```python
from build123d import *

# Parameters (mm, degrees)
EXTRUDE_1_DEPTH = 5
SKETCH_2_R      = 2.5
EXTRUDE_2_DEPTH = 8
SKETCH_3_R      = 3
EXTRUDE_3_DEPTH = 15
SKETCH_5_R      = 3.5
EXTRUDE_4_DEPTH = 2
SKETCH_4_W      = 0.25
SKETCH_4_H      = 0.7
SKETCH_4_W_2    = 1.323985747
SKETCH_4_H_2    = 1
CHAMFER_1_SIZE  = 0.2


with BuildPart() as part:
    # 草图1 → 拉伸1 (new body)
    with BuildSketch(Plane.XY):
        with BuildLine():
            Line((-2.633913438, 4.25), (2.633913438, 4.25))
            ThreePointArc((2.633913438, 4.25), (4.982386472, 0.419314968), (3.307189139, -3.75))
            Line((3.307189139, -3.75), (-3.307189139, -3.75))
            ThreePointArc((-3.307189139, -3.75), (-4.982386472, 0.419314968), (-2.633913438, 4.25))
        make_face()
    extrude(amount=EXTRUDE_1_DEPTH)

    # 草图2 → 拉伸2 (add)
    with BuildSketch(Plane.XY.offset(5)):
        Circle(SKETCH_2_R)
    extrude(amount=EXTRUDE_2_DEPTH)

    # 草图3 → 拉伸3 (add)
    with BuildSketch(Plane(origin=(0, 0, 0), x_dir=(-1, 0, 0), z_dir=(0, 0, -1))):
        with Locations(Location((0, 0, 0), (0, 0, 180))):
            Circle(SKETCH_3_R)
    extrude(amount=EXTRUDE_3_DEPTH)

    # 草图5 → 拉伸4 (add)
    with BuildSketch(Plane(origin=(0, 0, 0), x_dir=(-1, 0, 0), z_dir=(0, 0, -1))):
        with Locations(Location((0, 0, 0), (0, 0, 180))):
            Circle(SKETCH_5_R)
    extrude(amount=EXTRUDE_4_DEPTH)

    # 草图4 → 切除-旋转1 (revolve, cut)
    with BuildSketch(Plane(origin=(0, 0, 0), x_dir=(1, 0, 0), z_dir=(0, 1, 0))):
        with Locations((-2.875, 13.55)):
            Rectangle(SKETCH_4_W, SKETCH_4_H)
        with Locations((-2.661992874, -5.5)):
            Rectangle(SKETCH_4_W_2, SKETCH_4_H_2)
    revolve(axis=Axis((0, 0, -15), (0, 0, 1)), mode=Mode.SUBTRACT)

    # 倒角1
    chamfer_1_edges = [part.edges().sort_by_distance(p)[0] for p in [
        (-2.5, 0, 13),
        (-3, 0, -15),
    ]]
    chamfer(chamfer_1_edges, length=CHAMFER_1_SIZE)


solid = part.part
```
Read the model definition and answer for the solid it produces. Units are mm, in the model's axes. A direction names the side the tool comes from. Round coordinates to 2 decimals unless told otherwise and drop trailing zeros. Write each loop counter-clockwise with the first axis right and the second up, starting at its lowest first coordinate (ties: lowest second). Pieces come first, ordered by that corner, then holes. Notation, with made-up numbers: (-35.5, -20) - (12.5, -20) arc R24 cw to (12.5, 18) - close; hole circle Ø8 at (58, 58.5). An arc over 180 degrees is marked (long way). One line per item, written item: value.
Q1. This flat-tipped pin is pushed along its axis until it touches: P1, Ø2, axis at x = -2.5, y = 3, coming from the -Z side. Where does it stop, or does it pass through?
The answers:
P1: stops at z = -14.89
Q2. Find section C-C (z = 2.75). Determine the outline of the cut face in (x, y), and give its area (3 significant figures).
The answers:
outline: (-3.31, -3.75) - (3.31, -3.75) arc R5 ccw to (2.63, 4.25) - (-2.63, 4.25) arc R5 ccw to start
area: 70.2 mm2
Q3. Straight lines are drawn through the part: line 1 (Z direction, x = -1.75, y = 1.25); line 2 (Z direction, x = 3.5, y = -2.75); line 3 (Y direction, x = -4.25, z = 0.25). For each, find the intervals that lie inside material, in ascending order. Write a range as from..to.
The answers:
line 1: z = -15..5, 6..13
line 2: z = 0..5
line 3: y = -2.63..2.63
Q4. Which of the six approach directions +Z, -Z, +X, -X, +Y, -Y give full straight-line access (tool end or side, diameter ignored) to faces 1 (the cylindrical face through (0.26, -1.983, 5.493)), 2 (the cylindrical face through (3.233, 1.341, -0.986)), 3 (the cylindrical face through (-0.54, -2.44, 9.35))?
The answers:
face 1: none
face 2: -Z
face 3: +Z
Q5. Find section D-D (y = 3.75). Determine the outline of the cut face in (x, z), and give its area (3 significant figures).
The answers:
outline: (-3.31, 0) - (3.31, 0) - (3.31, 5) - (-3.31, 5) - close
area: 33.1 mm2
